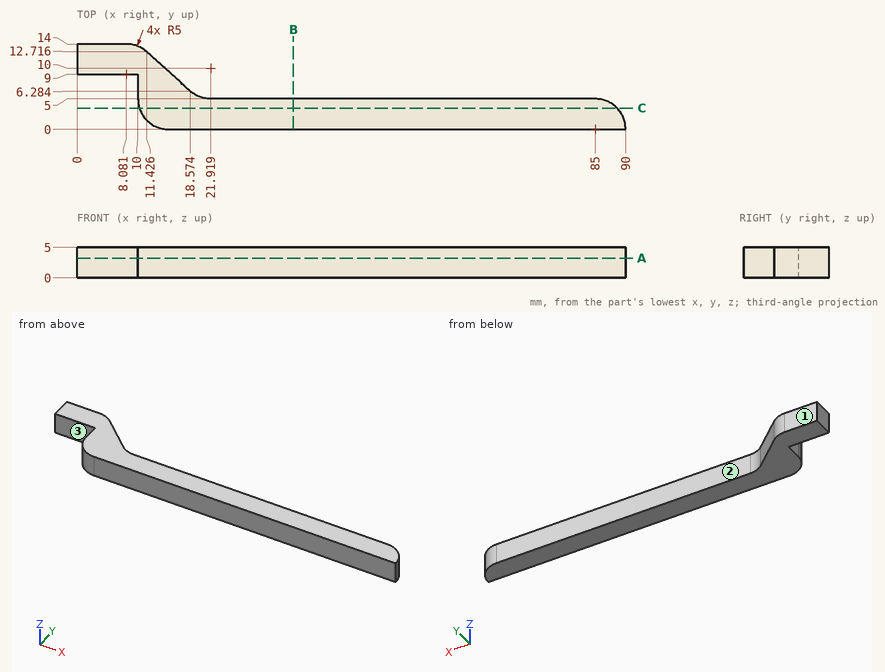
Source: three-view drawing plus pictorial views. Frame: mm from the lowest corner of the part. A direction names the side the tool comes from. Coordinates: 2 decimals unless noted, no trailing zeros. Write each loop counter-clockwise with the first axis right and the second up, starting at its lowest first coordinate (ties: lowest second). Pieces come first, ordered by that corner, then holes. Notation, with made-up numbers: (36.5, 8.5) - (80.5, 8.5) arc R27 cw to (80.5, 34.5) - close; hole circle Ø10 at (64.5, 35.5). An arc over 180 degrees is marked (long way). Return JSON: item names as keys, results as strings.
Item 1: Reachability of the marked faces 1, 2 and 3 from +Z, -Z, +X, -X, +Y, -Y: full face, straight path, thin tool, end or side. Return the list, or none.
Completed:
{"face 1": "+Z, -Z, +X, -X, +Y", "face 2": "+Z, -Z, +X, +Y", "face 3": "+Z, -Z, -X, -Y"}
Item 2: Pin query (flat end, axial travel): pin 1 Ø1.5 at (x, z) = (6, 3) entering from -Y; pin 2 Ø1.5 at (x, z) = (56, 4.5) entering from +Y. Return the tip coordinate at first contact, or that it passes through.
Completed:
{"pin 1": "stops at y = 9", "pin 2": "stops at y = 5"}
Item 3: Section query A-A (z = 3.25). Output: boundary loops of the cut face in (x, y).
Completed:
{"outline": "(0, 9) - (10, 9) - (10, 5) arc R5 ccw to (15, 0) - (90, 0) arc R5 ccw to (85, 5) - (21.92, 5) arc R5 cw to (18.57, 6.28) - (11.43, 12.72) arc R5 ccw to (8.08, 14) - (0, 14) - close"}
Item 4: Section query C-C (y = 3.5). Output: boundary loops of the cut face in (x, z), and give its area (3 significant figures).
Completed:
{"outline": "(10.23, 0) - (88.57, 0) - (88.57, 5) - (10.23, 5) - close", "area": "392 mm2"}
Item 5: Section query B-B (x = 35.5). Output: boundary loops of the cut face in (y, z), and give its area (3 significant figures).
Completed:
{"outline": "(0, 0) - (5, 0) - (5, 5) - (0, 5) - close", "area": "25.0 mm2"}
Item 6: Line query: L1, parallel to Y at x = 61.5, z = 3.7; L2, parallel to Y at x = 6, z = 1.1; L3, parallel to X at y = 2.5, z = 2.7. Output: solid intervals per line, ascending.
Completed:
{"L1": "y = 0 to 5", "L2": "y = 9 to 14", "L3": "x = 10.67 to 89.33"}
